Here's how the part is built. I have some questions about the finished solid (model axes, mm). Face numbers are marked on the shaded views. A direction names the side the tool comes from. Round coordinates to 2 decimals unless told otherwise and drop trailing zeros. Order: outer loops, then holes, each group sorted by start corner. A loop starts at its lowest first (then second) coordinate and runs counter-clockwise, first axis right, second up. Notation, with made-up numbers: (55.25, -34) -> (68.25, -34) arc R6 ccw to (68.25, -26) -> close; hole circle Ø10 at (39, 20). An arc over 180 degrees is marked (long way). Use a Markdown table: item, result. Add a question column.
(1) On a 3-axis mill with a long thin cutter (end or side, diameter ignored), from which of +Z, -Z, +X, -X, +Y, -Y can I reach the whole of each face in a straight line? I mean the marked faces 5 and 6. Say none if no direction works.
(2) If I drill on probe 1 along Y at (x, z) = (0, 14.7); probe 2 along Z at (x, y) = (-2.25, 3.75); probe 3 along Y at (x, z) = (-1.5, 17), over which ranges is the centre line in solid material (lowest first)?
(3) I want a section at A-A, the plane x = 0. Please give me the cut outline in (y, z), then the cut area to 3 significant figures.
(4) Thinking about a two-plate mould opening in X: for the marked faces 1, 2, 3 and 4, which applies, pulls with the +X half, pulls with the -X half, needs draft (parallel to the pull), parting line crosses it, or undercut?
(5) I'm going to push a flat-ended pin straight in: P1, Ø4, axis at x = -1, y = 0.5, coming from the -Z side. Where does the tip first touch, or does it pass through?
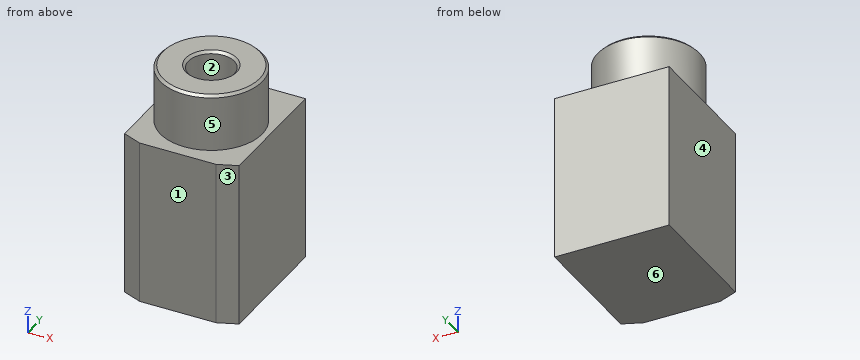
from build123d import *

# Parameters (mm, degrees)
F1_DEPTH = 13
F2_R     = 4
F2_R_2   = 1.8
F3_DEPTH = 4.5
F4_SIZE  = 0.2


with BuildPart() as f1:
    # F0 (on Top) → F1 (new body)
    with BuildSketch(Plane.XY):
        Polygon((4.5, 5.5), (0, 5.5), (-4.5, 5.5), (-4.5, -4.4), (-3, -5), (0, -5), (3, -5), (4.5, -4.4), align=None)
    extrude(amount=F1_DEPTH)

    # F2 (on face) → F3 (join)
    with BuildSketch(Plane.XY.offset(13)):
        Circle(F2_R)
        Circle(F2_R_2, mode=Mode.SUBTRACT)
    extrude(amount=F3_DEPTH)

    # F4
    f4_edges = [f1.edges().sort_by_distance(p)[0] for p in [
        (-4, 0, 17.5),
        (-1.8, 0, 17.5),
    ]]
    chamfer(f4_edges, length=F4_SIZE)


solid = f1.part
Taken from the geometry:
| question | item | result |
|---|---|---|
| 1 | face 5 | +Z |
| 1 | face 6 | -Z, +X, -X, +Y, -Y |
| 2 | probe 1 | y = -4 to -1.8, 1.8 to 4 |
| 2 | probe 2 | z = 0 to 13 |
| 2 | probe 3 | y = -3.71 to -0.99, 0.99 to 3.71 |
| 3 | outline | (-5, 0) -> (5.5, 0) -> (5.5, 13) -> (4, 13) -> (4, 17.3) -> (3.8, 17.5) -> (2, 17.5) -> (1.8, 17.3) -> (1.8, 13) -> (-1.8, 13) -> (-1.8, 17.3) -> (-2, 17.5) -> (-3.8, 17.5) -> (-4, 17.3) -> (-4, 13) -> (-5, 13) -> close |
| 3 | area | 156 mm2 |
| 4 | face 1 | needs draft |
| 4 | face 2 | undercut |
| 4 | face 3 | pulls with the +X half |
| 4 | face 4 | pulls with the -X half |
| 5 | P1 | stops at z = 0 |
